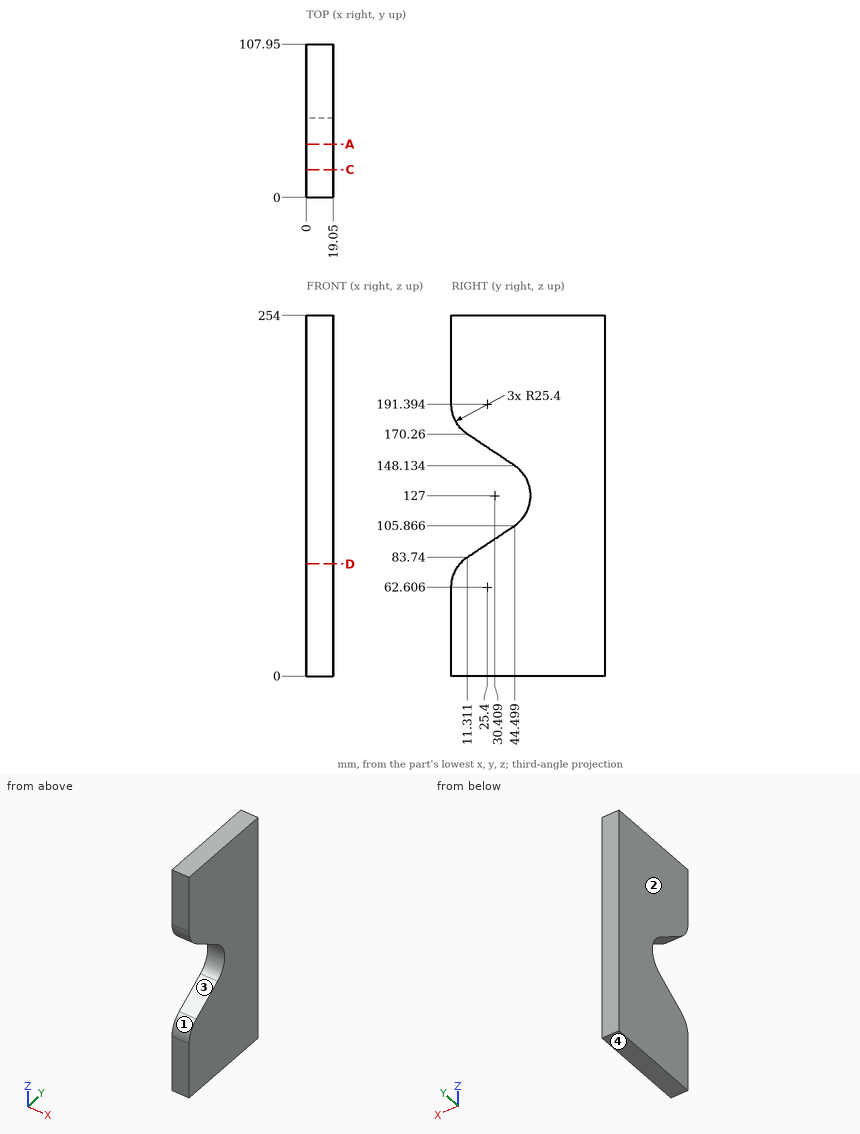
For this review, use the dimensioned drawing (mm, ordinates from the lowest corner) and the shaded views. Round coordinates to 2 decimals unless told otherwise and drop trailing zeros. Write each loop counter-clockwise with the first axis right and the second up, starting at its lowest first coordinate (ties: lowest second). Pieces come first, ordered by that corner, then holes. Notation, with made-up numbers: (79, 21.25) - (127, 21.25) arc R27 ccw to (127, 48.25) - close; hole circle Ø4 at (18.5, -27). An arc over 180 degrees is marked (long way). One line per item, written item: value. Start each with the question number.
1. The part is to be moulded in two halves that separate along Z. For the marked faces 1, 2, 3 and 4, say which applies: released by +Z, released by -Z, zero draft, split by the parting line, or undercut.
2. Consider section D-D on z = 79. Write out the cut boundary in (x, y).
3. To check wall thickness, follow L1, parallel to Z at x = 18.25, y = 34 (1 decimal); L2, parallel to Z at x = 3.75, y = 32 (1 decimal); L3, parallel to Y at x = 10.75, z = 80. State the ranges of each line that lie inside material, in increasing order. Write a range as from..to.
4. Consider section A-A on y = 37.5. Write out the cut boundary in (x, z).
5. Clearance check with a flat-ended pin moving along its axis: P1, Ø8, axis at x = 14.5, y = 52.5, coming from the -Z side. State where the tip first meets the part, or that it passes through.
6. Consider section C-C on y = 19.5. Write out the cut boundary in (x, z), and give its area (3 significant figures).
Checks:
1. face 1: undercut
1. face 2: zero draft
1. face 3: undercut
1. face 4: released by -Z
2. outline: (0, 6) - (19.05, 6) - (19.05, 107.95) - (0, 107.95) - close
3. L1: z = 0..98.9, 155.1..254
3. L2: z = 0..97.5, 156.5..254
3. L3: y = 6.89..107.95
4. outline: (0, 0) - (19.05, 0) - (19.05, 101.2) - (0, 101.2) - close; (0, 152.8) - (19.05, 152.8) - (19.05, 254) - (0, 254) - close
5. P1: stops at z = 0
6. outline: (0, 0) - (19.05, 0) - (19.05, 89.2) - (0, 89.2) - close; (0, 164.8) - (19.05, 164.8) - (19.05, 254) - (0, 254) - close
6. area: 3,400 mm^2
